Design review of the part built by this model. Coordinates are the model's own, in mm. Face numbers are marked on the shaded views. Give positions to 0.01 mm unless a question says otherwise; leave off trailing zeros. Write each loop counter-clockwise with the first axis right and the second up, starting at its lowest first coordinate (ties: lowest second). Pieces come first, ordered by that corner, then holes. Notation, with made-up numbers: (71.25, 50) -> (85.25, 50) arc R27 ccw to (85.25, 86) -> close; hole circle Ø4 at (-16, -29.5). An arc over 180 degrees is marked (long way). Return JSON: item names as keys, results as strings. Group by question number.
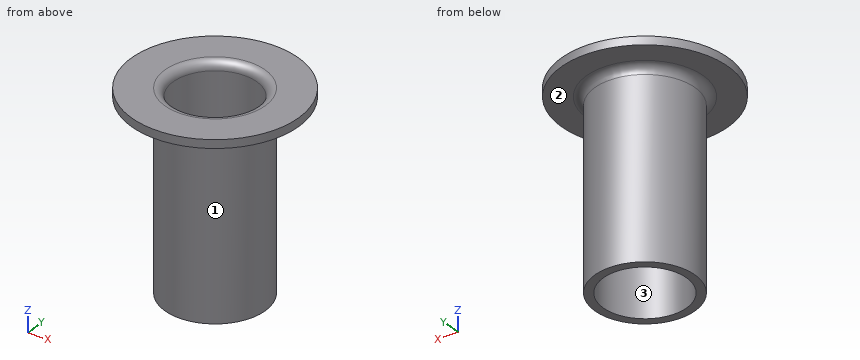
Autodesk Inventor part; units mm, degrees
ref_plane "YZ Plane" through (0, 0, 0) normal (1, 0, 0) x (0, 1, 0)
ref_plane "XZ Plane" through (0, 0, 0) normal (0, 1, 0) x (-1, 0, 0)
ref_plane "XY Plane" through (0, 0, 0) normal (0, 0, 1) x (1, 0, 0)
sketch "Sketch1" plane through (0, 0, 0) normal (0, 0, 1) x (1, 0, 0)
  circle A0 centre (0, 0) radius 2.5
  circle A1 centre (0, 0) radius 1.25
  circle A2 centre (0, 0) radius 1.5
  dimension "d0" = 5
  dimension "d1" = 2.5
  dimension "d2" = 3
extrude "Extrusion1" add sketch "Sketch1" against normal blind 0.25 contours A0
extrude "Extrusion2" add sketch "Sketch1" against normal blind 5.8 contours A2
fillet "Fillet1" radius 0.25 1 edges at (-1.25, 0, 0)
fillet "Fillet2" radius 0.25 1 edges at (-1.5, 0, -0.25)
properties part number "Standard Servo Brass Sleeve"
Q1. For L1, parallel to Y at x = 0, z = -2.45; L2, parallel to Z at x = -0.85, y = -1.9; L3, parallel to Y at x = 0.6, z = -2.65, list the stretches that pass through material, from the lowest coordinate up. Write a range as from..to.
Q2. Mouldability with a two-part tool opening along X and no side actions: class the marked faces 1, 2 and 3 as +X half, -X half, draft (parallel to the pull), parting line (faces both ways), or undercut.
Q3. Take a section at A-A, the plane y = 0. Give the boundary of the cut face in (x, z).
Q4. Insertion check: pin 1 (3 mm diameter, centred on x = -1.5, z = -2.5, fed in from -Y); pin 2 (2 mm diameter, centred on x = -0.5, z = -2, fed in from +Y); pin 3 (3 mm diameter, centred on y = 0.5, z = -4, fed in from +X). Each pin has a flat end and moves straight along its axis. Give the tip position at first contact, or say it passes through.
Q5. Take a section at C-C, the plane z = -3.6. Give the boundary of the cut face in (x, y).
Q6. Take a section at D-D, the plane y = -2. Give the boundary of the cut face in (x, z).
Final values:
{
 "1": {"L1": "y = -1.5..-1.25, 1.25..1.5", "L2": "z = -0.25..0", "L3": "y = -1.37..-1.1, 1.1..1.37"},
 "2": {"face 1": "parting line", "face 2": "draft", "face 3": "undercut"},
 "3": {"outline": "(-2.5, -0.25) -> (-1.75, -0.25) arc R0.25 cw to (-1.5, -0.5) -> (-1.5, -5.8) -> (-1.25, -5.8) -> (-1.25, -0.25) arc R0.25 ccw to (-1.5, 0) -> (-2.5, 0) -> close; (1.25, -5.8) -> (1.5, -5.8) -> (1.5, -0.5) arc R0.25 cw to (1.75, -0.25) -> (2.5, -0.25) -> (2.5, 0) -> (1.5, 0) arc R0.25 ccw to (1.25, -0.25) -> close"},
 "4": {"pin 1": "stops at y = -1.5", "pin 2": "stops at y = 1.5", "pin 3": "stops at x = 1.5"},
 "5": {"outline": "circle Ø3 at (0, 0); hole circle Ø2.5 at (0, 0)"},
 "6": {"outline": "(-1.5, -0.25) -> (1.5, -0.25) -> (1.5, 0) -> (-1.5, 0) -> close"}
}
